from build123d import *

# Parameters (mm, degrees)
SKETCH2_W           = 174.75062189439555
SKETCH2_H           = 55.00000000000001
BOSS_EXTRUDE1_DEPTH = 100
FILLET1_ANGLE       = 171.711787


with BuildPart() as part:
    # Sketch2 → Boss-Extrude1 (new body)
    with BuildSketch(Plane(origin=(0, 0, 0), x_dir=(0, 0, -1), z_dir=(1, 0, 0))):
        with Locations((87.37531094719778, 27.500000000000004)):
            Rectangle(SKETCH2_W, SKETCH2_H)
        with BuildLine():
            Line((0, 0), (0, 55.00000000000001))
            ThreePointArc((0, 55.00000000000001), (-45.24937810560445, 5.000000000000011), (5.51e-15, -45))
            Line((5.51e-15, -45), (0, 0))
        make_face()
    extrude(amount=BOSS_EXTRUDE1_DEPTH)

    # Fillet1: read off the stored shape, not the designer's step
    # Fillet1 outline → Fillet1 (revolve, cut)
    with BuildSketch(Plane(origin=(0, 5, -5), x_dir=(0, 0.998988212638407, 0.04497278076260073), z_dir=(0, 0.04497278076260073, -0.998988212638407))):
        with BuildLine():
            ThreePointArc((50.249378106, 0.1987375), (50.19116924, 0.058208866), (50.050640606, 0))
            Line((50.050640606, 0), (50.249378106, 0))
            Line((50.249378106, 0), (50.249378106, 0.1987375))
        make_face()
        with BuildLine():
            ThreePointArc((50.050640606, 100), (50.19116924, 99.941791134), (50.249378106, 99.8012625))
            Line((50.249378106, 99.8012625), (50.249378106, 100))
            Line((50.249378106, 100), (50.050640606, 100))
        make_face()
    revolve(axis=Axis((0, 5, -5), (1, 0, 0)), revolution_arc=FILLET1_ANGLE, mode=Mode.SUBTRACT)


solid = part.part
Part model, mm, in its own coordinate system. Coordinates: 2 decimals unless noted, no trailing zeros. Loops run counter-clockwise (first coordinate to the right, second up) from the corner with the lowest first, then second, coordinate; pieces in that order, holes last. Notation, with made-up numbers: M 55.5,-31.75 L 75.5,-31.75 A18 ccw 75.5,-3.75 Z; hole C -14.5,55 d5. An arc over 180 degrees is marked long. Use a Markdown table: item, result. Add a question column.
Q1. Pin check, flat tips, straight feed: P1, Ø10, axis at x = 48.5, y = -26.5, coming from the +Z side; P2, Ø10, axis at x = 63, y = -30, coming from the -Z side; P3, Ø10, axis at x = 82, z = -38, coming from the -Y side. Stop position of each tip, or through.
Q2. Cut at A-A (x = 76.5). Write the cut outline in (y, z), and give its area (3 significant figures).
Q3. Cut at B-B (z = -14.5). Write the cut outline in (x, y), and give its area (3 significant figures).
Q4. Mould opens along Z. For faces 1 (the flat face through (49, 0, -86)), 2 (the cylindrical face through (49.3, 6.03, 45.24)), 3 (the flat face through (49, -23, 0)) say: +Z half, -Z half, draft (parallel to the pull), parting line (faces both ways), or undercut.
Q5. Probe L1, parallel to Y at x = 59, z = -151.5; L2, parallel to Z at x = 80, y = 9; L3, parallel to Z at x = 85.5, y = 7. List the from-to ranges inside material, lowest first.
Worked out:
| question | item | result |
|---|---|---|
| 1 | P1 | stops at z = 37.69 |
| 1 | P2 | stops at z = 0 |
| 1 | P3 | stops at y = 0 |
| 2 | outline | M -45,0 L 0,0 L 0,-174.75 L 55,-174.75 L 55,0 A50.25 ccw Z |
| 2 | area | 13,100 mm2 |
| 3 | outline | M 0,0 L 100,0 L 100,55 L 0,55 Z |
| 3 | area | 5,500 mm2 |
| 4 | face 1 | draft |
| 4 | face 2 | +Z half |
| 4 | face 3 | -Z half |
| 5 | L1 | y = 0 to 55 |
| 5 | L2 | z = -174.75 to 45.09 |
| 5 | L3 | z = -174.75 to 45.21 |
